from build123d import *

# Parameters (mm, degrees)
F0_W        = 100
F0_H        = 100
F1_DEPTH    = 390
F2_T        = -2.5
F3_R        = 5
F4_DEPTH    = 2000
F5_T1_DEPTH = 595.7346390373
F6_W        = 95
F6_H        = 2.5
F7_DEPTH    = 59.6


# Not quite as in the source:
# - a fillet or chamfer that OpenCascade refuses, or shapes differently, is made with other operations: its cross-section is extruded or revolved along the edge and cut away or added


with BuildPart() as f1:
    # F0 (on Top) → F1 (new body)
    with BuildSketch(Plane.XY):
        with Locations((50, 50)):
            Rectangle(F0_W, F0_H)
    extrude(amount=F1_DEPTH)

    # F2
    f2_openings = [f1.faces().sort_by_distance(p)[0] for p in [
        (50, 100, 195),
    ]]
    offset(amount=F2_T, openings=f2_openings)

    # F3 (on face) → F4 (cut)
    with BuildSketch(Plane(origin=(0, 0, 0), x_dir=(1, 0, 0), z_dir=(0, 0, -1))):
        with Locations((50, -89.3280655146)):
            Circle(F3_R)
    extrude(amount=-F4_DEPTH, mode=Mode.SUBTRACT)

    # F5: chamfer of 40 on 2 edges, made by hand

    # F5_s2 → F5_t1 (cut)
    with BuildSketch(Plane.XY.offset(-102.8673195186)):
        Polygon((0, 60), (40, 100), (0, 100), align=None)
        Polygon((60, 100), (100, 60), (100, 100), align=None)
    extrude(amount=F5_T1_DEPTH, mode=Mode.SUBTRACT)

    # F6 (on face) → F7 (join)
    with BuildSketch(Plane(origin=(0, 2.5, 0), x_dir=(-1, 0, 0), z_dir=(0, 1, 0))):
        with Locations((-50, 328.2103848457)):
            Rectangle(F6_W, F6_H)
        with Locations((-50, 257.6169383526)):
            Rectangle(F6_W, F6_H)
        with Locations((-50, 151.1440885067)):
            Rectangle(F6_W, F6_H)
    extrude(amount=F7_DEPTH)


solid = f1.part
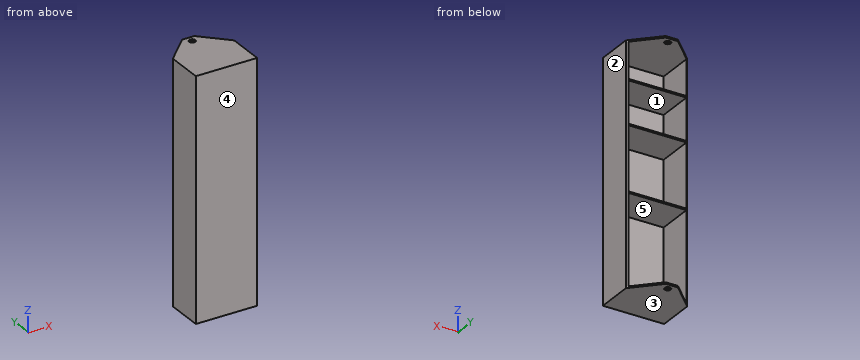
For this review, take the finished solid that the model builds, in its own axes (mm). Face numbers are marked on the shaded views. A direction names the side the tool comes from. Round coordinates to 2 decimals unless told otherwise and drop trailing zeros. Write each loop counter-clockwise with the first axis right and the second up, starting at its lowest first coordinate (ties: lowest second). Pieces come first, ordered by that corner, then holes. Notation, with made-up numbers: (-31.5, 49) - (20.5, 49) arc R25 cw to (20.5, 67) - close; hole circle Ø11 at (42, 77). An arc over 180 degrees is marked (long way). Write item = value, one per line. Start each with the question number.
1. For the marked faces 4 and 5, list the 3-axis set-ups (+Z, -Z, +X, -X, +Y, -Y) from which the entire face can be reached by the end or side of a thin tool; tool diameter is ignored.
2. Consider section B-B on x = 50. State the section outline as (y, z) points.
3. Wall thickness on L1, parallel to Z at x = 64, y = 61; L2, parallel to X at y = 13, z = 224.5; L3, parallel to Y at x = 50, z = 388.3: over which ranges is each line inside the solid? List them lowest first.
4. Consider section A-A on y = 79. State the section outline as (x, z) points.
5. For pin 1 Ø1 at (x, z) = (28, 294.5) entering from +Y; pin 2 Ø5 at (y, z) = (29, 217) entering from -X; pin 3 Ø2 at (x, z) = (57.5, 258) entering from +Y, all flat-tipped, find the tip position at first contact; note any pin that passes through.
6. Consider section C-C on z = 309.5. State the section outline as (x, y) points.
7. Draft analysis for pull direction Z (two halves, no side actions). For the marked faces 1, 2 and 3, state which applies: released by +Z, released by -Z, zero draft, split by the parting line, or undercut.
8. Consider section D-D on x = 65. State the section outline as (y, z) points.
Evaluation:
q1.face_4 = +Z, -Z, +X, -X, -Y
q1.face_5 = +Y
q2.outline = (0, 0) - (84.33, 0) - (84.33, 2.5) - (2.5, 2.5) - (2.5, 149.89) - (62.1, 149.89) - (62.1, 152.39) - (2.5, 152.39) - (2.5, 256.37) - (62.1, 256.37) - (62.1, 258.87) - (2.5, 258.87) - (2.5, 326.96) - (62.1, 326.96) - (62.1, 329.46) - (2.5, 329.46) - (2.5, 387.5) - (84.33, 387.5) - (84.33, 390) - (0, 390) - close; (94.33, 0) - (100, 0) - (100, 2.5) - (94.33, 2.5) - close; (94.33, 387.5) - (100, 387.5) - (100, 390) - (94.33, 390) - close
q3.L1 = 0 to 2.5, 149.89 to 152.39, 256.37 to 258.87, 326.96 to 329.46, 387.5 to 390
q3.L2 = 0 to 2.5, 97.5 to 100
q3.L3 = 0 to 84.33, 94.33 to 100
q4.outline = (19, 0) - (81, 0) - (81, 2.5) - (19, 2.5) - close; (19, 387.5) - (81, 387.5) - (81, 390) - (19, 390) - close
q5.pin_1 = 2.5
q5.pin_2 = 0
q5.pin_3 = 62.1
q6.outline = (0, 0) - (100, 0) - (100, 60) - (97.5, 62.5) - (97.5, 2.5) - (2.5, 2.5) - (2.5, 62.5) - (0, 60) - close
q7.face_1 = undercut
q7.face_2 = zero draft
q7.face_3 = released by -Z
q8.outline = (0, 0) - (95, 0) - (95, 2.5) - (2.5, 2.5) - (2.5, 149.89) - (62.1, 149.89) - (62.1, 152.39) - (2.5, 152.39) - (2.5, 256.37) - (62.1, 256.37) - (62.1, 258.87) - (2.5, 258.87) - (2.5, 326.96) - (62.1, 326.96) - (62.1, 329.46) - (2.5, 329.46) - (2.5, 387.5) - (95, 387.5) - (95, 390) - (0, 390) - close
